from build123d import *

# Parameters (mm, degrees)
SKETCH1_R               = 5.357495
SKETCH1_R_2             = 2.182495
RAISER_DEPTH            = 4.7625
RAISER_2_DEPTH          = 4.7625
SKETCH3_R               = 2.182495
PLATFORM_DEPTH          = 3.175
WALLS_DEPTH             = 76.2
SKETCH9_W               = 31.75
SKETCH9_H               = 3.302
BOSS_EXTRUDE4_DEPTH     = 25.4
BOSS_EXTRUDE5_DEPTH     = 31.75
BOSS_EXTRUDE6_DEPTH     = 3.175
SKETCH13_R              = 1.585905821
CUT_EXTRUDE1_DEPTH      = 3.175
SKETCH14_W              = 22.86
SKETCH14_H              = 38.1
CUT_EXTRUDE2_DEPTH      = 2.54
SKETCH16_W              = 22.86
SKETCH16_H              = 26.817011057
CUT_EXTRUDE3_DEPTH      = 5080
SKETCH17_W              = 20.32
SKETCH17_H              = 38.1
CUT_EXTRUDE4_DEPTH      = 2.54
SKETCH18_W              = 20.32
SKETCH18_H              = 25.4
CUT_EXTRUDE5_DEPTH      = 8.9375
SKETCH21_R              = 23.434999297
CUT_EXTRUDE6_DEPTH      = 5.7625
CUT_EXTRUDE7_DEPTH      = 77.2
CUT_EXTRUDE7_DEPTH_BACK = 4.175
SKETCH23_W              = 0.822798121
SKETCH23_H              = 25.4
CUT_EXTRUDE8_DEPTH      = 22.448562342
CUT_EXTRUDE8_DEPTH_BACK = 58.926437658
CUT_EXTRUDE9_DEPTH      = 1
CUT_EXTRUDE9_DEPTH_BACK = 80.375


with BuildPart() as part:
    # Sketch1 → Raiser (new body)
    with BuildSketch(Plane(origin=(0, 0, 0), x_dir=(1, 0, 0), z_dir=(0, 1, 0))):
        with Locations((-24.991443565, 0)):
            Circle(SKETCH1_R)
        with Locations((-24.991443565, 0)):
            Circle(SKETCH1_R_2, mode=Mode.SUBTRACT)
    extrude(amount=RAISER_DEPTH)



with BuildPart() as body_2:
    # Sketch1 → Raiser 2 (new body)
    with BuildSketch(Plane(origin=(0, 0, 0), x_dir=(1, 0, 0), z_dir=(0, 1, 0))):
        with Locations((46.849916435, 0)):
            Circle(SKETCH1_R)
        with Locations((46.849916435, 0)):
            Circle(SKETCH1_R_2, mode=Mode.SUBTRACT)
    extrude(amount=RAISER_2_DEPTH)


with BuildPart() as part_1:
    add(part.part)

    add(body_2.part)  # Platform merges body 2
    # Sketch3 → Platform (add)
    with BuildSketch(Plane(origin=(0, 4.7625, 0), x_dir=(1, 0, 0), z_dir=(0, 1, 0))):
        with BuildLine():
            Line((-32.611443565, 8.933868965), (-32.611443565, -17.883142092))
            ThreePointArc((-32.611443565, -17.883142092), (27.714936864, -31.227394881), (74.666125822, 8.933868965))
            Line((74.666125822, 8.933868965), (-32.611443565, 8.933868965))
        make_face()
        with Locations((-24.991443565, 0)):
            Circle(SKETCH3_R, mode=Mode.SUBTRACT)
        with Locations((46.849916435, 0)):
            Circle(SKETCH3_R, mode=Mode.SUBTRACT)
    extrude(amount=PLATFORM_DEPTH)

    # Sketch7 → Walls (add)
    with BuildSketch(Plane(origin=(0, 7.9375, 0), x_dir=(1, 0, 0), z_dir=(0, 1, 0))):
        with BuildLine():
            Line((74.666125822, 8.933868965), (-32.611443565, 8.933868965))
            Line((-32.611443565, 8.933868965), (-32.611443565, 6.393868965))
            Line((-32.611443565, 6.393868965), (-30.071443565, 6.393868965))
            Line((-30.071443565, 6.393868965), (73.529899121, 6.393868965))
            ThreePointArc((73.529899121, 6.393868965), (74.110777774, 7.65815862), (74.666125822, 8.933868965))
        make_face()
    extrude(amount=WALLS_DEPTH)

    # Sketch9 → Boss-Extrude4 (add)
    with BuildSketch(Plane(origin=(0, 0, -8.933868965), x_dir=(-1, 0, 0), z_dir=(0, 0, -1))):
        with Locations((-58.791125822, 61.037937658)):
            Rectangle(SKETCH9_W, SKETCH9_H)
    extrude(amount=BOSS_EXTRUDE4_DEPTH)

    # Sketch10 → Boss-Extrude5 (add)
    with BuildSketch(Plane.ZY.offset(-42.916125822)):
        Polygon((-34.333868965, 59.386937658), (-8.933868965, 51.890363409), (-8.933868965, 59.386937658), align=None)
    extrude(amount=-BOSS_EXTRUDE5_DEPTH)

    # Sketch12 → Boss-Extrude6 (add)
    with BuildSketch(Plane(origin=(0, 84.1375, 0), x_dir=(1, 0, 0), z_dir=(0, 1, 0))):
        with BuildLine():
            Line((-32.611443565, 6.393868965), (-32.611443565, -17.883142092))
            ThreePointArc((-32.611443565, -17.883142092), (-20.588039105, -25.701496657), (-7.211443565, -30.874079638))
            Line((-7.211443565, -30.874079638), (-7.211443565, 6.393868965))
            Line((-7.211443565, 6.393868965), (-32.611443565, 6.393868965))
        make_face()
    extrude(amount=-BOSS_EXTRUDE6_DEPTH)

    # Sketch13 → Cut-Extrude1 (cut)
    with BuildSketch(Plane(origin=(0, 84.1375, 0), x_dir=(1, 0, 0), z_dir=(0, 1, 0))):
        with Locations((-11.081791728, -2.408517057)):
            Circle(SKETCH13_R)
        with Locations((-11.081791728, -18.283517057)):
            Circle(SKETCH13_R)
    extrude(amount=-CUT_EXTRUDE1_DEPTH, mode=Mode.SUBTRACT)

    # Sketch14 → Cut-Extrude2 (cut)
    with BuildSketch(Plane.XY.offset(-6.393868965)):
        with Locations((-21.181443565, 26.9875)):
            Rectangle(SKETCH14_W, SKETCH14_H)
    extrude(amount=-CUT_EXTRUDE2_DEPTH, mode=Mode.SUBTRACT)

    # Sketch16 → Cut-Extrude3 (cut)
    with BuildSketch(Plane(origin=(0, 7.9375, 0), x_dir=(1, 0, 0), z_dir=(0, 1, 0))):
        with Locations((-21.181443565, -4.474636563)):
            Rectangle(SKETCH16_W, SKETCH16_H)
    extrude(amount=-CUT_EXTRUDE3_DEPTH, mode=Mode.SUBTRACT)

    # Sketch17 → Cut-Extrude4 (cut)
    with BuildSketch(Plane.XY.offset(-6.393868965)):
        with Locations((10.929236435, 26.9875)):
            Rectangle(SKETCH17_W, SKETCH17_H)
    extrude(amount=-CUT_EXTRUDE4_DEPTH, mode=Mode.SUBTRACT)

    # Sketch18 → Cut-Extrude5 (cut, through all)
    with BuildSketch(Plane(origin=(0, 7.9375, 0), x_dir=(1, 0, 0), z_dir=(0, 1, 0))):
        with Locations((10.929236435, -3.766131035)):
            Rectangle(SKETCH18_W, SKETCH18_H)
    extrude(amount=-CUT_EXTRUDE5_DEPTH, mode=Mode.SUBTRACT)

    # Sketch21 → Cut-Extrude6 (cut, through all)
    with BuildSketch(Plane.XZ.offset(-4.7625)):
        with Locations((35.627803811, 7.157128957)):
            Circle(SKETCH21_R)
    extrude(amount=CUT_EXTRUDE6_DEPTH, mode=Mode.SUBTRACT)

    # Sketch22 → Cut-Extrude7 (cut, two sides)
    with BuildSketch(Plane(origin=(0, 7.9375, 0), x_dir=(1, 0, 0), z_dir=(0, 1, 0))) as cut_extrude7_sk:
        with BuildLine():
            ThreePointArc((72.686340907, 6.393868965), (26.479298711, -30.742030079), (-31.389645862, -17.883142092))
            Line((-31.389645862, -17.883142092), (-32.611443565, -17.883142092))
            ThreePointArc((-32.611443565, -17.883142092), (26.361801078, -31.551234168), (73.529899121, 6.393868965))
            Line((73.529899121, 6.393868965), (72.686340907, 6.393868965))
        make_face()
        with BuildLine():
            ThreePointArc((73.505417676, 8.171868965), (73.102235438, 7.279940859), (72.686340907, 6.393868965))
            Line((72.686340907, 6.393868965), (73.529899121, 6.393868965))
            ThreePointArc((73.529899121, 6.393868965), (74.110777774, 7.65815862), (74.666125822, 8.933868965))
            Line((74.666125822, 8.933868965), (73.843327701, 8.933868965))
            Line((73.843327701, 8.933868965), (73.505417676, 8.171868965))
        make_face()
    extrude(amount=CUT_EXTRUDE7_DEPTH, mode=Mode.SUBTRACT)
    extrude(cut_extrude7_sk.sketch, amount=-CUT_EXTRUDE7_DEPTH_BACK, mode=Mode.SUBTRACT)

    # Sketch23 → Cut-Extrude8 (cut, two sides)
    with BuildSketch(Plane(origin=(0, 62.688937658, 0), x_dir=(1, 0, 0), z_dir=(0, 1, 0))) as cut_extrude8_sk:
        with Locations((74.254726761, 21.633868965)):
            Rectangle(SKETCH23_W, SKETCH23_H)
    extrude(amount=CUT_EXTRUDE8_DEPTH, mode=Mode.SUBTRACT)
    extrude(cut_extrude8_sk.sketch, amount=-CUT_EXTRUDE8_DEPTH_BACK, mode=Mode.SUBTRACT)

    # Sketch24 → Cut-Extrude9 (cut, two sides)
    with BuildSketch(Plane(origin=(0, 84.1375, 0), x_dir=(1, 0, 0), z_dir=(0, 1, 0))) as cut_extrude9_sk:
        Polygon((-32.611443565, -16.922161086), (-32.611443565, -17.883142092), (-31.389645862, -17.883142092), align=None)
    extrude(amount=CUT_EXTRUDE9_DEPTH, mode=Mode.SUBTRACT)
    extrude(cut_extrude9_sk.sketch, amount=-CUT_EXTRUDE9_DEPTH_BACK, mode=Mode.SUBTRACT)


solid = part_1.part
Could you check a few things on this model? Use its own coordinates, in mm. A direction names the side the tool comes from. Give positions to 0.01 mm unless a question says otherwise; leave off trailing zeros. Order: outer loops, then holes, each group sorted by start corner. A loop starts at its lowest first (then second) coordinate and runs counter-clockwise, first axis right, second up. Notation, with made-up numbers: M 2.25,39 L 53.25,39 A11 ccw 53.25,51 Z; hole C 46.5,-39.75 d4. An arc over 180 degrees is marked long. One line per question, with ' | ' between items.
1. For faces 1 (the face through (-9.751, 16, -7)), 2 (the face through (-21, 46.038, -8)), 3 (the face through (-12.251, 82.572, 1.337)), 4 (the face through (42.916, 59, -19)), 5 (the face through (11, 46.038, -8)), which set-ups out of +Z, -Z, +X, -X, +Y, -Y let a thin tool reach every point of the face, with its end or its side?
Results:
face 1: -Z, -X, -Y | face 2: +Z, -Z, -X, -Y | face 3: +Y | face 4: -Z, -X, +Y, -Y | face 5: +Z, -Z, -Y
2. I want a section at C-C (z = 8.5). List the corners of the cut face in (x, y) for me.
Results:
outline: M -32.61,80.96 L -7.21,80.96 L -7.21,84.14 L -32.61,84.14 Z; M -9.75,4.76 L 0.77,4.76 L 0.77,7.94 L -9.75,7.94 Z; M 21.09,4.76 L 63.01,4.76 L 63.01,7.94 L 21.09,7.94 Z
3. We'd pull the mould along X, two halves only. Please class faces 6 (the face through (11, 6, 16.466)), 7 (the face through (73.843, 59, -19)), 8 (the face through (21.4, 43.9, -8.934)): +X half, -X half, draft (parallel to the pull), parting line (faces both ways), or undercut.
Results:
face 6: undercut | face 7: +X half | face 8: draft
4. If I drill on line 1 (X direction, y = 6.55, z = 0); line 2 (Z direction, x = 11, y = 59); line 3 (Y direction, x = 8.5, z = 24), over which ranges is the centre line in solid material (lowest first)?
Results:
line 1: -9.75 to 0.77, 21.09 to 44.67, 49.03 to 69.2 | line 2: -8.93 to -6.39 | line 3: 4.76 to 7.94
5. I want a section at D-D (y = 67). List the corners of the cut face in (x, z) for me.
Results:
outline: M -32.61,-8.93 L 73.84,-8.93 L 73.51,-8.17 A68.45 ccw 72.69,-6.39 L -32.61,-6.39 Z
6. I'm going to push flat-ended pins straight in: pin 1 (1.3 mm diameter, centred on x = -18, z = -8, fed in from -Y); pin 2 (3 mm diameter, centred on x = -11.08, z = 2.41, fed in from +Y); pin 3 (6 mm diameter, centred on x = 2, y = 32.5, fed in from +Z); pin 4 (12.5 mm diameter, centred on y = 27.5, z = 5, fed in from -X). Where does each tip first touch, or does it pass through?
Results:
pin 1: y = 46.04 | pin 2: y = 7.94 | pin 3: z = -6.39 | pin 4: through
7. I want a section at B-B (x = 8). List the corners of the cut face in (y, z) for me, and give its area (3 significant figures).
Results:
outline: M 4.76,16.47 L 7.94,16.47 L 7.94,32.47 L 4.76,32.47 Z; M 46.04,-8.93 L 84.14,-8.93 L 84.14,-6.39 L 46.04,-6.39 Z | area: 148 mm²
8. I want a section at A-A (z = 25.5). List the corners of the cut face in (x, y) for me, and give its area (3 significant figures).
Results:
outline: M -19.29,4.76 L 41.15,4.76 L 41.15,7.94 L -19.29,7.94 Z; M -19.29,80.96 L -7.21,80.96 L -7.21,84.14 L -19.29,84.14 Z | area: 230 mm²
